```python
from build123d import *

# Parameters (mm, degrees)
SKETCH4_R           = 60
BOSS_EXTRUDE2_DEPTH = 32
CUT_EXTRUDE1_DEPTH  = 12
CUT_EXTRUDE2_DEPTH  = 12
SKETCH4_18_R        = 5
CUT_EXTRUDE6_DEPTH  = 12
SKETCH4_19_R        = 5
CUT_EXTRUDE7_DEPTH  = 40
SKETCH4_20_R        = 5
CUT_EXTRUDE8_DEPTH  = 40
SKETCH4_21_R        = 5
CUT_EXTRUDE9_DEPTH  = 40
SKETCH4_22_R        = 5
CUT_EXTRUDE10_DEPTH = 40
SKETCH4_23_R        = 5
CUT_EXTRUDE11_DEPTH = 40


with BuildPart() as part:
    # Sketch4 → Boss-Extrude2 (new body)
    with BuildSketch(Plane(origin=(0, 0, 0), x_dir=(1, 0, 0), z_dir=(0, 1, 0))):
        with Locations(Location((0, 0, 0), (0, 0, 270))):
            Circle(SKETCH4_R)
    extrude(amount=BOSS_EXTRUDE2_DEPTH)

    # Sketch4_4 → Cut-Extrude1 (cut)
    with BuildSketch(Plane(origin=(0, 0, 0), x_dir=(1, 0, 0), z_dir=(0, 1, 0))):
        with BuildLine():
            ThreePointArc((24.954792471, 43.222968452), (0, 49.909584942), (-24.954792471, 43.222968452))
            ThreePointArc((-24.954792471, 43.222968452), (-26.052868682, 39.124892241), (-21.954792471, 38.026816029))
            ThreePointArc((-21.954792471, 38.026816029), (0, 43.909584942), (21.954792471, 38.026816029))
            ThreePointArc((21.954792471, 38.026816029), (26.052868682, 39.124892241), (24.954792471, 43.222968452))
        make_face()
    extrude(amount=CUT_EXTRUDE1_DEPTH, mode=Mode.SUBTRACT)

    # Sketch4_5 → Cut-Extrude2 (cut)
    with BuildSketch(Plane(origin=(0, 0, 0), x_dir=(1, 0, 0), z_dir=(0, 1, 0))):
        with BuildLine():
            ThreePointArc((24.954792471, -43.222968452), (0, -49.909584942), (-24.954792471, -43.222968452))
            ThreePointArc((-24.954792471, -43.222968452), (-26.052868682, -39.124892241), (-21.954792471, -38.026816029))
            ThreePointArc((-21.954792471, -38.026816029), (0, -43.909584942), (21.954792471, -38.026816029))
            ThreePointArc((21.954792471, -38.026816029), (26.052868682, -39.124892241), (24.954792471, -43.222968452))
        make_face()
    extrude(amount=CUT_EXTRUDE2_DEPTH, mode=Mode.SUBTRACT)

    # Sketch4_18 → Cut-Extrude6 (cut)
    with BuildSketch(Plane(origin=(0, 0, 0), x_dir=(1, 0, 0), z_dir=(0, 1, 0))):
        with BuildLine():
            ThreePointArc((60, 0), (59.74389008, 5.537833341), (58.97774673, 11.028390213))
            Line((58.97774673, 11.028390213), (12, 11.028390213))
            Line((12, 11.028390213), (12, 25))
            ThreePointArc((12, 25), (0, 37), (-12, 25))
            Line((-12, 25), (-12, 11.028390213))
            Line((-12, 11.028390213), (-58.97774673, 11.028390213))
            ThreePointArc((-58.97774673, 11.028390213), (-59.997958043, -0.495005778), (-58.787753827, -12))
            Line((-58.787753827, -12), (-12, -12))
            Line((-12, -12), (-12, -25))
            ThreePointArc((-12, -25), (0, -37), (12, -25))
            Line((12, -25), (12, -12))
            Line((12, -12), (58.787753827, -12))
            ThreePointArc((58.787753827, -12), (58.795548236, -11.961751865), (58.80331776, -11.923498667))
            ThreePointArc((58.80331776, -11.923498667), (59.700079839, -5.99169986), (60, 0))
        make_face()
        with Locations(Location((0, -30, 0), (0, 0, 270))):
            Circle(SKETCH4_18_R, mode=Mode.SUBTRACT)
        with Locations(Location((-40, 0, 0), (0, 0, 270))):
            Circle(SKETCH4_18_R, mode=Mode.SUBTRACT)
        with BuildLine():
            ThreePointArc((0, 5), (3.535533906, 3.535533906), (5, 0))
            ThreePointArc((5, 0), (-3.535533906, -3.535533906), (0, 5))
        make_face(mode=Mode.SUBTRACT)
        with Locations(Location((40, 0, 0), (0, 0, 270))):
            Circle(SKETCH4_18_R, mode=Mode.SUBTRACT)
        with Locations(Location((0, 30, 0), (0, 0, 270))):
            Circle(SKETCH4_18_R, mode=Mode.SUBTRACT)
    extrude(amount=CUT_EXTRUDE6_DEPTH, mode=Mode.SUBTRACT)

    # Sketch4_19 → Cut-Extrude7 (cut)
    with BuildSketch(Plane(origin=(0, 0, 0), x_dir=(1, 0, 0), z_dir=(0, 1, 0))):
        with Locations(Location((0, -30, 0), (0, 0, 270))):
            Circle(SKETCH4_19_R)
    extrude(amount=CUT_EXTRUDE7_DEPTH, mode=Mode.SUBTRACT)

    # Sketch4_20 → Cut-Extrude8 (cut)
    with BuildSketch(Plane(origin=(0, 0, 0), x_dir=(1, 0, 0), z_dir=(0, 1, 0))):
        with Locations(Location((-40, 0, 0), (0, 0, 270))):
            Circle(SKETCH4_20_R)
    extrude(amount=CUT_EXTRUDE8_DEPTH, mode=Mode.SUBTRACT)

    # Sketch4_21 → Cut-Extrude9 (cut)
    with BuildSketch(Plane(origin=(0, 0, 0), x_dir=(1, 0, 0), z_dir=(0, 1, 0))):
        with Locations(Location((0, 0, 0), (0, 0, 270))):
            Circle(SKETCH4_21_R)
    extrude(amount=CUT_EXTRUDE9_DEPTH, mode=Mode.SUBTRACT)

    # Sketch4_22 → Cut-Extrude10 (cut)
    with BuildSketch(Plane(origin=(0, 0, 0), x_dir=(1, 0, 0), z_dir=(0, 1, 0))):
        with Locations(Location((40, 0, 0), (0, 0, 270))):
            Circle(SKETCH4_22_R)
    extrude(amount=CUT_EXTRUDE10_DEPTH, mode=Mode.SUBTRACT)

    # Sketch4_23 → Cut-Extrude11 (cut)
    with BuildSketch(Plane(origin=(0, 0, 0), x_dir=(1, 0, 0), z_dir=(0, 1, 0))):
        with Locations(Location((0, 30, 0), (0, 0, 270))):
            Circle(SKETCH4_23_R)
    extrude(amount=CUT_EXTRUDE11_DEPTH, mode=Mode.SUBTRACT)


solid = part.part
```
For this review, take the finished solid that the model builds, in its own axes (mm). A direction names the side the tool comes from. Give positions to 0.01 mm unless a question says otherwise; leave off trailing zeros. Write each loop counter-clockwise with the first axis right and the second up, starting at its lowest first coordinate (ties: lowest second). Pieces come first, ordered by that corner, then holes. Notation, with made-up numbers: M 66.25,-26.75 L 101.25,-26.75 A29 cw 101.25,-1.75 Z; hole C 23.25,82 d9. An arc over 180 degrees is marked long. One line per item, written item: value.
1) The part is to be moulded in two halves that separate along Z. For faces 1 (the cylindrical face through (0, 6, 37)), 2 (the flat face through (1, 0, -41)), say which applies: +Z half, -Z half, draft (parallel to the pull), parting line (faces both ways), or undercut.
Results are:
face 1: undercut
face 2: draft
2) Take a section at A-A, the plane y = 3.5. Write out the cut boundary in (x, z), then the cut area to 3 significant figures.
Results are:
outline: M -58.98,-11.03 A60 ccw 58.98,-11.03 L 12,-11.03 L 12,-25 A12 cw -12,-25 L -12,-11.03 Z; M -58.79,12 L -12,12 L -12,25 A12 cw 12,25 L 12,12 L 58.79,12 A60 ccw Z; hole M -24.95,-43.22 A49.91 ccw 24.95,-43.22 A3 ccw 21.95,-38.03 A43.91 cw -21.95,-38.03 A3 ccw Z; hole M -24.95,43.22 A3 ccw -21.95,38.03 A43.91 cw 21.95,38.03 A3 ccw 24.95,43.22 A49.91 ccw Z
area: 6,820 mm²
3) For line 1 (X direction, y = 19, z = 0); line 2 (Z direction, x = 0, y = 16.75); line 3 (X direction, y = 6.5, z = -15), list the stretches that pass through material, from the lowest coordinate up. Write a range as from..to.
Results are:
line 1: x = -60..-45, -35..-5, 5..35, 45..60
line 2: z = -60..-35, -25..-5, 5..25, 35..60
line 3: x = -58.09..-12, 12..58.09
4) Take a section at C-C, the plane x = 37. Write out the cut boundary in (y, z).
Results are:
outline: M 0,-47.23 L 32,-47.23 L 32,-4 L 12,-4 L 12,-11.03 L 0,-11.03 Z; M 0,12 L 12,12 L 12,4 L 32,4 L 32,47.23 L 0,47.23 Z
5) Take a section at B-B, the plane z = 0. Write out the cut boundary in (x, y), then the cut area to 3 significant figures.
Results are:
outline: M -60,12 L -45,12 L -45,32 L -60,32 Z; M -35,12 L -5,12 L -5,32 L -35,32 Z; M 5,12 L 35,12 L 35,32 L 5,32 Z; M 45,12 L 60,12 L 60,32 L 45,32 Z
area: 1,800 mm²
6) For faces 3 (the flat face through (35, 6, 12)), 4 (the cylindrical face through (0, 22, -35)), 5 (the cylindrical face through (-0.32, 5.92, -43.91)), list the 3-axis set-ups (+Z, -Z, +X, -X, +Y, -Y) from which the entire face can be reached by the end or side of a thin tool; tool diameter is ignored.
Results are:
face 3: +X, -X, -Y
face 4: +Y, -Y
face 5: -Y
7) Take a section at D-D, the plane y = 27. Write out the cut boundary in (x, z).
Results are:
outline: C 0,0 d120; hole C -40,0 d10; hole C 0,-30 d10; hole C 0,0 d10; hole C 0,30 d10; hole C 40,0 d10
8) For P1, Ø6, axis at y = 3.5, z = 16, coming from the -X side; P2, Ø10, axis at x = -0.5, z = 20.5, coming from the -Y side; P3, Ø9.5, axis at y = 4, z = -19, coming from the -X side, all flat-tipped, find the tip position at first contact; note any pin that passes through.
Results are:
P1: stops at x = -58.57
P2: stops at y = 12
P3: stops at x = -58.28
